from build123d import *

# Parameters (mm, degrees)
F0_W     = 14.5
F0_H     = 9
F0_W_2   = 12.5
F0_H_2   = 7
F1_DEPTH = 2
F2_DEPTH = 1
F3_R     = 0.75
F4_DEPTH = 3.001
F5_W     = 14.5
F5_H     = 1.5
F6_DEPTH = 3.75
F7_R     = 1.05
F7_W     = 2
F7_H     = 9
F8_DEPTH = 1.5


with BuildPart() as f1:
    # F0 (on Top) → F1 (new body)
    with BuildSketch(Plane.XY):
        Rectangle(F0_W, F0_H)
        Rectangle(F0_W_2, F0_H_2, mode=Mode.SUBTRACT)
    extrude(amount=F1_DEPTH)

    # F0 (on Top) → F2 (join)
    with BuildSketch(Plane.XY):
        Rectangle(F0_W, F0_H)
        Rectangle(F0_W_2, F0_H_2, mode=Mode.SUBTRACT)
        Rectangle(F0_W_2, F0_H_2)
    extrude(amount=-F2_DEPTH)

    # F3 (on face) → F4 (cut, through all)
    with BuildSketch(Plane(origin=(0, 0, -1), x_dir=(1, 0, 0), z_dir=(0, 0, -1))):
        with Locations((-4, 1.5)):
            Circle(F3_R)
        with Locations((4, 1.5)):
            Circle(F3_R)
        with Locations((4, -1.5)):
            Circle(F3_R)
        with Locations((-4, -1.5)):
            Circle(F3_R)
    extrude(amount=-F4_DEPTH, mode=Mode.SUBTRACT)

    # F5 (on face) → F6 (join)
    with BuildSketch(Plane(origin=(0, 0, -1), x_dir=(1, 0, 0), z_dir=(0, 0, -1))):
        with Locations((0, 3.75)):
            Rectangle(F5_W, F5_H)
        with Locations((0, -3.75)):
            Rectangle(F5_W, F5_H)
    extrude(amount=F6_DEPTH)

    # F7 (on face) → F8 (join)
    with BuildSketch(Plane(origin=(0, 0, -4.75), x_dir=(1, 0, 0), z_dir=(0, 0, -1))):
        Polygon((-13, -1.8759706765), (-7.25, -4.5), (-7.25, 4.5), (-13, 1.8759706765), align=None)
        with Locations((-9.95, 0)):
            Circle(F7_R, mode=Mode.SUBTRACT)
        with Locations((-6.25, 0)):
            Rectangle(F7_W, F7_H)
    extrude(amount=-F8_DEPTH)


solid = f1.part
Part model, mm, in its own coordinate system. A direction names the side the tool comes from. Give positions to 0.01 mm unless a question says otherwise; leave off trailing zeros. Loops run counter-clockwise (first coordinate to the right, second up) from the corner with the lowest first, then second, coordinate; pieces in that order, holes last. Notation, with made-up numbers: M 57,-6.75 L 61,-6.75 A9 ccw 61,1.25 Z; hole C 83.25,73 d3. An arc over 180 degrees is marked long. Put each result on its own line as item: value. Start each with the question number.
1) Saw through at A-A (y = 1.5). List the corners of the cut face in (x, z), then the cut area to 3 significant figures.
2) Pull direction Z, two halves, no side cores. Call faces 1 (the flat face through (-7.25, 0, 0)), 2 (the flat face through (0, -4, 2)), 3 (the flat face through (-8, 0, -3.25)): +Z half, -Z half, draft (parallel to the pull), parting line (faces both ways), or undercut.
3) Saw through at D-D (x = -7). List the corners of the cut face in (y, z).
4) Probe probe 1 along Y at (x, z) = (-4, -0.35); probe 2 along X at (y, z) = (-1.5, -0.55); probe 3 along Y at (x, z) = (5.5, -2.5). List the from-to ranges inside material, lowest first.
5) Saw through at C-C (y = 0). List the corners of the cut face in (x, z), then the cut area to 3 significant figures.
6) Flat gauge pins, fed straight in: pin 1 (1.4 mm diameter, centred on x = -4, y = 1.5, fed in from +Z); pin 2 (1.7 mm diameter, centred on x = 4, y = -1.5, fed in from -Z); pin 3 (1.6 mm diameter, centred on y = 0, z = -0.5, fed in from -X); pin 4 (2 mm diameter, centred on y = -2.5, z = -2, fed in from +X). Where does each tip first touch, or does it go through?
7) Saw through at B-B (x = -4). List the corners of the cut face in (y, z), then the cut area to 4 significant figures.
8) 3-axis set-ups, long thin cutter, end or side, ignore diameter. For faces 4 (the flat face through (0, 0, 0)), 5 (the flat face through (-5.25, 0, -4)), 6 (the cylindrical face through (-4.55, 0.99, -0.51)): which of +Z, -Z, +X, -X, +Y, -Y reach the whole face in a straight line?
Numbers:
1. outline: M -13,-4.75 L -5.25,-4.75 L -5.25,-3.25 L -13,-3.25 Z; M -7.25,-1 L -4.75,-1 L -4.75,0 L -6.25,0 L -6.25,2 L -7.25,2 Z; M -3.25,-1 L 3.25,-1 L 3.25,0 L -3.25,0 Z; M 4.75,-1 L 7.25,-1 L 7.25,2 L 6.25,2 L 6.25,0 L 4.75,0 Z
1. area: 27.1 mm^2
2. face 1: draft
2. face 2: +Z half
2. face 3: undercut
3. outline: M -4.5,-4.75 L 4.5,-4.75 L 4.5,2 L -4.5,2 Z; hole M -3,-3.25 L 3,-3.25 L 3,-1 L -3,-1 Z
4. probe 1: -4.5 to -2.25, -0.75 to 0.75, 2.25 to 4.5
4. probe 2: -7.25 to -4.75, -3.25 to 3.25, 4.75 to 7.25
4. probe 3: -4.5 to -3, 3 to 4.5
5. outline: M -13,-4.75 L -11,-4.75 L -11,-3.25 L -13,-3.25 Z; M -8.9,-4.75 L -5.25,-4.75 L -5.25,-3.25 L -8.9,-3.25 Z; M -7.25,-1 L 7.25,-1 L 7.25,2 L 6.25,2 L 6.25,0 L -6.25,0 L -6.25,2 L -7.25,2 Z
5. area: 27.0 mm^2
6. pin 1: through
6. pin 2: z = -1
6. pin 3: x = -7.25
6. pin 4: x = 7.25
7. outline: M -4.5,-4.75 L -3,-4.75 L -3,-1 L -2.25,-1 L -2.25,0 L -3.5,0 L -3.5,2 L -4.5,2 Z; M -0.75,-1 L 0.75,-1 L 0.75,0 L -0.75,0 Z; M 2.25,-1 L 3,-1 L 3,-4.75 L 4.5,-4.75 L 4.5,2 L 3.5,2 L 3.5,0 L 2.25,0 Z
7. area: 21.25 mm^2
8. face 4: +Z
8. face 5: -Z, +X
8. face 6: +Z, -Z
